from build123d import *

# Parameters (mm, degrees)
PAD008_DEPTH         = 14
PAD008_DEPTH_BACK    = 5
POCKET006_DEPTH      = 30.001
POCKET006_DEPTH_BACK = 30.001
POCKET032_DEPTH      = 13.2908094213
PAD015_DEPTH         = 16
SKETCH026_W          = 0.7
SKETCH026_H          = 12
SKETCH027_W          = 0.7
SKETCH027_H          = 14
POCKET033_DEPTH      = 14.501
SKETCH037_R          = 1.65
POCKET034_DEPTH      = 14.001
PAD016_DEPTH         = 3
SKETCH036_W          = 6
SKETCH036_H          = 40
POCKET035_DEPTH      = 14.501
POCKET036_DEPTH      = 0.701
PAD017_DEPTH         = 10


with BuildPart() as part:
    # Sketch020 → Pad008 (new body, two sides)
    with BuildSketch(Plane.XY) as pad008_sk:
        with BuildLine():
            Line((26.6687054218, 29.981651204), (-27.3312945782, 23.981651204))
            ThreePointArc((-27.3312945782, 23.981651204), (-29.2353840537, 23.0007643871), (-30, 21))
            Line((-30, 21), (-30, -21))
            ThreePointArc((-30, -21), (-29.2353840537, -23.0007643871), (-27.3312945782, -23.981651204))
            Line((-27.3312945782, -23.981651204), (26.6687054218, -29.981651204))
            ThreePointArc((26.6687054218, -29.981651204), (29.0007643871, -29.2353840537), (30, -27))
            Line((30, -27), (30, 27))
            ThreePointArc((30, 27), (29.0007643871, 29.2353840537), (26.6687054218, 29.981651204))
        make_face()
    extrude(amount=PAD008_DEPTH)
    extrude(pad008_sk.sketch, amount=-PAD008_DEPTH_BACK)

    # Sketch021 → Pocket006 (cut, two sides)
    with BuildSketch(Plane.XZ) as pocket006_sk:
        Polygon((31, -6), (-31, -6), (-31, -0.466136402), (31, 10.466136402), align=None)
    extrude(amount=-POCKET006_DEPTH, mode=Mode.SUBTRACT)
    extrude(pocket006_sk.sketch, amount=POCKET006_DEPTH_BACK, mode=Mode.SUBTRACT)

    # Sketch040 → Pocket032 (cut, through all)
    with BuildSketch(Plane.XY.offset(13)):
        with BuildLine():
            Line((-25.2090569265, 20.276010124), (23.7909430735, 25.426117652))
            ThreePointArc((26, 23.4370738613), (25.3382612127, 24.9233635123), (23.7909430735, 25.426117652))
            Line((26, 23.4370738613), (26, 6.8045027298))
            Line((26, 6.8045027298), (17.6319194267, 3.7587704831))
            ThreePointArc((17.6319194267, 3.7587704831), (15, 0), (17.6319194267, -3.7587704831))
            Line((26, -6.8045027298), (17.6319194267, -3.7587704831))
            Line((26, -6.8045027298), (26, -23.4370738613))
            ThreePointArc((23.7909430735, -25.426117652), (25.3382612127, -24.9233635123), (26, -23.4370738613))
            Line((23.7909430735, -25.426117652), (-25.2090569265, -20.276010124))
            ThreePointArc((-27, -18.2869663333), (-26.486289651, -19.625227546), (-25.2090569265, -20.276010124))
            Line((-27, -18.2869663333), (-27, 18.2869663333))
            ThreePointArc((-25.2090569265, 20.276010124), (-26.486289651, 19.625227546), (-27, 18.2869663333))
        make_face()
    extrude(amount=-POCKET032_DEPTH, mode=Mode.SUBTRACT)

    # Sketch063 → Pad015 (join)
    with BuildSketch(Plane.XY.offset(-2.5)):
        with BuildLine():
            Line((15.5, 21), (15.5, 24.5547044207))
            Line((15.5, 24.5547044207), (8.5, 23.8189747738))
            Line((8.5, 21), (8.5, 23.8189747738))
            ThreePointArc((8.5, 21), (12, 17.5), (15.5, 21))
        make_face()
        with BuildLine():
            Line((8.5, -23.8189747738), (15.5, -24.5547044207))
            Line((15.5, -24.5547044207), (15.5, -21))
            ThreePointArc((15.5, -21), (12, -17.5), (8.5, -21))
            Line((8.5, -23.8189747738), (8.5, -21))
        make_face()
        with BuildLine():
            ThreePointArc((-25, 16), (-22.3826908751, 17.5338168788), (-22.4416970255, 20.5668713701))
            Line((-22.4416970255, 20.5668713701), (-26.5090569265, 20.1393746182))
            ThreePointArc((-26.5090569265, 20.1393746182), (-27.786289651, 19.4885920402), (-28.3, 18.1503308274))
            Line((-28.3, 16), (-28.3, 18.1503308274))
            Line((-25, 16), (-28.3, 16))
        make_face()
        with BuildLine():
            ThreePointArc((-22.4416970255, -20.5668713701), (-22.3826908751, -17.5338168788), (-25, -16))
            Line((-28.3, -16), (-25, -16))
            Line((-28.3, -18.1503308274), (-28.3, -16))
            ThreePointArc((-28.3, -18.1503308274), (-27.786289651, -19.4885920402), (-26.5090569265, -20.1393746182))
            Line((-22.4416970255, -20.5668713701), (-26.5090569265, -20.1393746182))
        make_face()
    extrude(amount=PAD015_DEPTH)

    # Sketch026 → Groove (revolve, cut)
    with BuildSketch(Plane.XZ.offset(21)):
        with Locations((12.35, 2.8)):
            Rectangle(SKETCH026_W, SKETCH026_H)
    groove = revolve(axis=Axis((12, -21, 8.8), (0, 0, -1)), mode=Mode.SUBTRACT)

    # Sketch027 → Groove004 (revolve, cut)
    with BuildSketch(Plane.XZ.offset(19)):
        with Locations((-25.35, 3.5)):
            Rectangle(SKETCH027_W, SKETCH027_H)
    groove004 = revolve(axis=Axis((-25, -19, -17.5), (0, 0, 1)), mode=Mode.SUBTRACT)

    # Mirrored013: Groove, Groove004 across XZ
    add(groove.mirror(Plane.XZ), mode=Mode.SUBTRACT)
    add(groove004.mirror(Plane.XZ), mode=Mode.SUBTRACT)

    # Sketch057 → Pocket033 (cut, through all)
    with BuildSketch(Plane.XY.offset(12)):
        with BuildLine():
            Line((21.9, -1.6743157806), (21.9, 1.6743157806))
            Line((21.9, 1.6743157806), (15.9010990338, 5.1377828683))
            ThreePointArc((15.9010990338, 5.1377828683), (13, 0), (15.9010990338, -5.1377828683))
            Line((15.9010990338, -5.1377828683), (21.9, -1.6743157806))
        make_face()
    extrude(amount=-POCKET033_DEPTH, mode=Mode.SUBTRACT)

    # Sketch037 → Pocket034 (cut, through all)
    with BuildSketch(Plane.XY):
        with Locations((19, 0)):
            Circle(SKETCH037_R)
    extrude(amount=POCKET034_DEPTH, mode=Mode.SUBTRACT)

    # Sketch039 → Pad016 (join)
    with BuildSketch(Plane.XY.offset(8.6)):
        Polygon((28.9, -11.85), (28.9, 11.85), (30, 14.8722251614), (30, -14.8722251614), align=None)
    extrude(amount=PAD016_DEPTH)

    # SubtractivePipe: sweep along a path in Sketch020
    with BuildLine(Plane.XY) as subtractivepipe_path:
        Line((26.6687054218, 29.981651204), (-27.3312945782, 23.981651204))
        ThreePointArc((-27.3312945782, 23.981651204), (-29.2353840537, 23.0007643871), (-30, 21))
        Line((-30, 21), (-30, -21))
        ThreePointArc((-30, -21), (-29.2353840537, -23.0007643871), (-27.3312945782, -23.981651204))
        Line((-27.3312945782, -23.981651204), (26.6687054218, -29.981651204))
        ThreePointArc((26.6687054218, -29.981651204), (29.0007643871, -29.2353840537), (30, -27))
        Line((30, -27), (30, 27))
        ThreePointArc((30, 27), (29.0007643871, 29.2353840537), (26.6687054218, 29.981651204))
    # Sketch035 → SubtractivePipe (sweep, cut)
    with BuildSketch(Plane.XZ):
        Polygon((28.5995849236, 14), (30, 14), (30, 12), align=None)
    sweep(path=subtractivepipe_path.line, mode=Mode.SUBTRACT)

    # Sketch036 → Pocket035 (cut, through all)
    with BuildSketch(Plane.XY.offset(12)):
        with Locations((26, 0)):
            Rectangle(SKETCH036_W, SKETCH036_H)
    extrude(amount=-POCKET035_DEPTH, mode=Mode.SUBTRACT)

    # Sketch054 → Pocket036 (cut, through all)
    with BuildSketch(Plane.YZ.offset(-29.3)):
        with BuildLine():
            Line((-4, 2), (4, 2))
            ThreePointArc((7, -1), (6.1213203436, 1.1213203436), (4, 2))
            Line((7, -1), (7, -3))
            ThreePointArc((4, -6), (6.1213203436, -5.1213203436), (7, -3))
            Line((4, -6), (-4, -6))
            ThreePointArc((-7, -3), (-6.1213203436, -5.1213203436), (-4, -6))
            Line((-7, -3), (-7, -1))
            ThreePointArc((-4, 2), (-6.1213203436, 1.1213203436), (-7, -1))
        make_face()
    extrude(amount=-POCKET036_DEPTH, mode=Mode.SUBTRACT)

    # Sketch064 → Pad017 (join)
    with BuildSketch(Plane.XY.offset(3.3)):
        with BuildLine():
            Line((1.4095389312, 20.486969785), (2.4646015442, 23.3857304905))
            Line((2.4646015442, 23.3857304905), (-2.2829835631, 22.8867391884))
            Line((-1.4095389312, 20.486969785), (-2.2829835631, 22.8867391884))
            ThreePointArc((-1.4095389312, 20.486969785), (0, 19.5), (1.4095389312, 20.486969785))
        make_face()
    pad017 = extrude(amount=PAD017_DEPTH)

    # Mirrored014: Pad017 across XZ
    add(pad017.mirror(Plane.XZ))

    # SubtractivePipe002: sweep along a path in Sketch023
    with BuildLine(Plane(origin=(0, 0, 4), x_dir=(0.984807753, 0, 0.1736481777), z_dir=(-0.1736481777, 0, 0.984807753))) as subtractivepipe002_path:
        Line((-26.343872324, 21.9802268076), (25.656127676, 27.9802268076))
        ThreePointArc((25.656127676, 27.9802268076), (27.996043966, 27.2396000728), (29, 25))
        Line((29, 25), (29, -25))
        ThreePointArc((29, -25), (27.996043966, -27.2396000728), (25.656127676, -27.9802268076))
        Line((25.656127676, -27.9802268076), (-26.343872324, -21.9802268076))
        ThreePointArc((-26.343872324, -21.9802268076), (-28.2396000728, -20.996043966), (-29, -19))
        Line((-29, -19), (-29, 19))
        ThreePointArc((-29, 19), (-28.2396000728, 20.996043966), (-26.343872324, 21.9802268076))
    # Sketch025 → SubtractivePipe002 (sweep, cut)
    with BuildSketch(Plane.XZ):
        Polygon((28.0823303903, 11.7415342162), (27.5746170843, 8.8621489747), (29.5442325904, 9.20944533), align=None)
    sweep(path=subtractivepipe002_path.line, mode=Mode.SUBTRACT)


solid = part.part
For this review, take the finished solid that the model builds, in its own axes (mm). A direction names the side the tool comes from. Give positions to 0.01 mm unless a question says otherwise; leave off trailing zeros. Loops run counter-clockwise (first coordinate to the right, second up) from the corner with the lowest first, then second, coordinate; pieces in that order, holes last.
Item 1: Tool access review of faces 1 (the flat face through (0.12, 23.14, 4.12)), 2 (the flat face through (-1.84, 21.67, 8.08)), 3 (the cylindrical face through (-29.65, 5.88, 1.34)), 4 (the flat face through (29.25, -0.12, 9.72)): name each direction out of +Z, -Z, +X, -X, +Y, -Y from which nothing blocks a thin tool from reaching the whole face with its end or side.
Item 2: Take a section at C-C, the plane y = 8.5. State the section outline as (x, z) points, and give its area (3 significant figures).
Item 3: Take a section at D-D, the plane x = -18. State the section outline as (y, z) points.
Item 4: Draft analysis for pull direction X (two halves, no side actions). For faces 5 (the flat face through (-0.631, 26.234, 13.014)), 6 (the flat face through (-27, 0, 7)), 7 (the flat face through (13, -21, -2.5)), state which applies: +X half, -X half, draft (parallel to the pull), parting line (faces both ways), or undercut.
Item 5: Take a section at A-A, the plane y = 0. State the section outline as (x, z) points.
Item 6: For line 1 along X through (y, z) = (-19, 9); line 2 along X through (y, z) = (-15.5, 11.75); line 3 along Y through (x, z) = (23, 12.25), list the stretches that pass through material, from the lowest coordinate up.
Item 7: Take a section at B-B, the plane x = 19. State the section outline as (y, z) points, and give its area (3 significant figures).
Item 8: Insertion check: pin 1 (0.5 mm diameter, centred on x = 29.5, y = 0.5, fed in from -Z); pin 2 (1.1 mm diameter, centred on y = -23, z = 4.5, fed in from +X); pin 3 (0.8 mm diameter, centred on y = -22, z = 7.5, fed in from -X); pin 4 (2.5 mm diameter, centred on x = 19, y = 0, fed in from +Z). Each pin has a flat end and moves straight along its axis. Give the tip position at first contact, or say it passes through.
Calculated:
1. face 1: -Z, +Y
1. face 2: -Z
1. face 3: -Z, -X
1. face 4: none
2. outline: (-30, -0.29) - (-29.36, -0.18) - (-29.04, 1.67) - (-28.1, 0.05) - (-27, 0.24) - (-27, 13) - (26, 13) - (26, 12) - (29, 12) - (29, 10.15) - (29.54, 9.21) - (29, 9.11) - (29, 8.6) - (30, 8.6) - (30, 12) - (28.6, 14) - (-28.6, 14) - (-30, 12) - close
2. area: 102 mm2
3. outline: (-25.02, 1.83) - (-23.58, 1.83) - (-22.97, 3.62) - (-22.29, 1.83) - (-21.03, 1.83) - (-21.03, 13) - (21.03, 13) - (21.03, 1.83) - (22.29, 1.83) - (22.97, 3.62) - (23.58, 1.83) - (25.02, 1.83) - (25.02, 12) - (23.61, 14) - (-23.61, 14) - (-25.02, 12) - close
4. face 5: -X half
4. face 6: undercut
4. face 7: draft
5. outline: (-30, 2) - (-29.3, 2) - (-29.3, 0.18) - (-29.04, 1.67) - (-28.1, 0.05) - (-27, 0.24) - (-27, 13) - (15, 13) - (15, 12) - (17.35, 12) - (17.35, 14) - (-28.6, 14) - (-30, 12) - close; (20.65, 12) - (21.9, 12) - (21.9, 8.86) - (23, 9.06) - (23, 12) - (29, 12) - (29, 10.15) - (29.54, 9.21) - (29, 9.11) - (29, 8.6) - (30, 8.6) - (30, 12) - (28.6, 14) - (20.65, 14) - close
6. line 1: x = -30 to -25.7, -24.3 to -22, 9.13 to 14.87
6. line 2: x = -30 to -27, 29 to 30
6. line 3: y = -29.4 to -25.34, -5.71 to 5.71, 25.34 to 29.4
7. outline: (-29.13, 8.35) - (-27.91, 8.35) - (-27.3, 10.14) - (-26.62, 8.35) - (-24.92, 8.35) - (-24.92, 13) - (-4.26, 13) - (-4.26, 8.35) - (-3.35, 8.35) - (-3.35, 12) - (-1.65, 12) - (-1.65, 14) - (-27.72, 14) - (-29.13, 12) - close; (1.65, 12) - (3.35, 12) - (3.35, 8.35) - (4.26, 8.35) - (4.26, 13) - (24.92, 13) - (24.92, 8.35) - (26.62, 8.35) - (27.3, 10.14) - (27.91, 8.35) - (29.13, 8.35) - (29.13, 12) - (27.72, 14) - (1.65, 14) - close
7. area: 101 mm2
8. pin 1: stops at z = 8.6
8. pin 2: stops at x = 15.5
8. pin 3: stops at x = -29.94
8. pin 4: passes through
